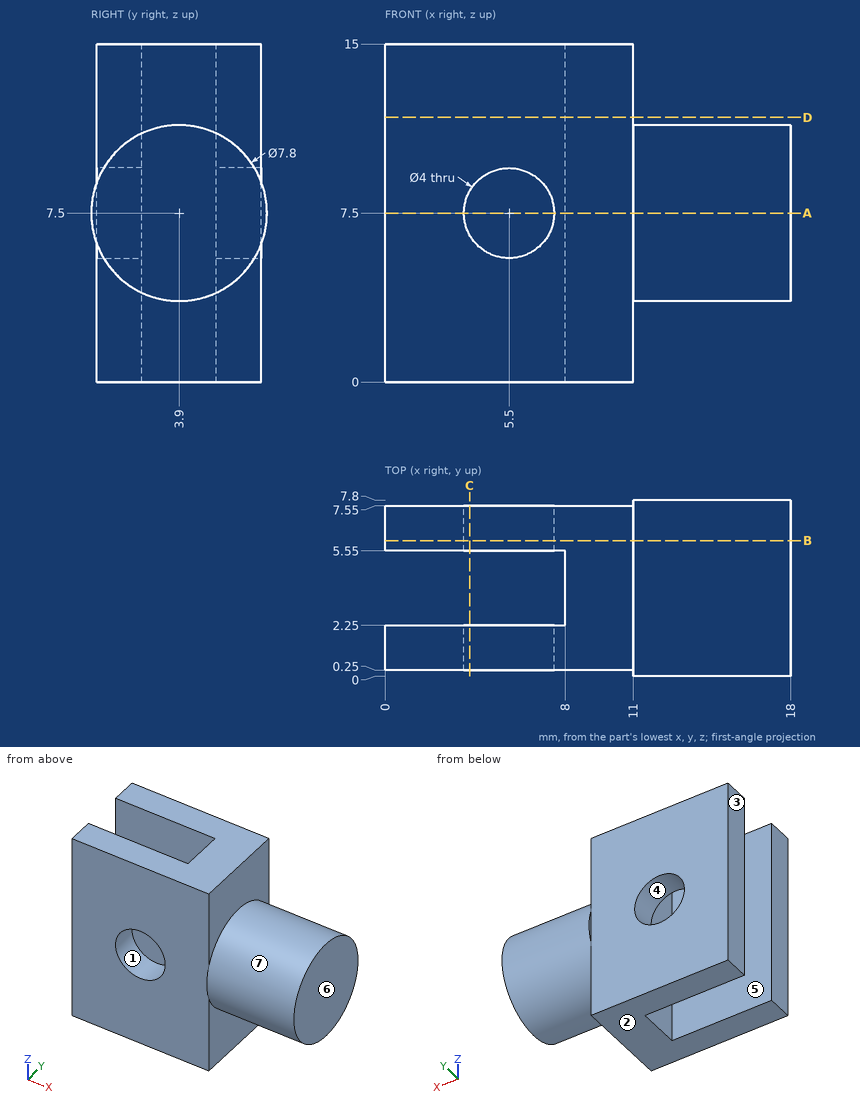
Source: three-view drawing plus pictorial views. Frame: mm from the lowest corner of the part. A direction names the side the tool comes from. Coordinates: 2 decimals unless noted, no trailing zeros. Order: outer loops, then holes, each group sorted by start corner. A loop starts at its lowest first (then second) coordinate and runs counter-clockwise, first axis right, second up. Notation, with made-up numbers: M 69.5,47 L 75.5,47 A16 cw 75.5,78 Z; hole C 3.5,85.5 d3. An arc over 180 degrees is marked long. One line per question, with ' | ' between items. Start each with the question number.
Item 1: Ray query, probe 1 along X at (y, z) = (7.05, 7.5); probe 2 along Y at (x, z) = (5.5, 4.75); probe 3 along X at (y, z) = (7, 1.25). Return the intervals inside material, ascending. Write a range as [from, to].
Item 2: Set-up query: the marked faces 5, 6 and 7. Return all of +Z, -Z, +X, -X, +Y, -Y with unobstructed straight access to the full face (end or side cutting, diameter ignored); none if empty.
Item 3: Cut plane C-C, the plane x = 3.75. Return the cut outline in (y, z), then the cut area to 3 significant figures.
Item 4: Pin query (flat end, axial travel): pin 1 Ø5.5 at (x, z) = (5.5, 11) entering from -Y; pin 2 Ø1.6 at (y, z) = (3.5, 5) entering from -X; pin 3 Ø4.5 at (x, z) = (5.5, 7.5) entering from +Y. Return the tip coordinate at first contact, or that it passes through.
Item 5: Cut plane A-A, the plane z = 7.5. Return the cut outline in (x, y), then the cut area to 3 significant figures.
Item 6: Cut plane D-D, the plane z = 11.75. Return the cut outline in (x, y), then the cut area to 3 significant figures.
Item 7: Draft query along Z for the marked faces 1, 2, 3 and 4. Return one class per face: released by +Z, released by -Z, zero draft, split by the parting line, or undercut.
Item 8: Cut plane B-B, the plane y = 6. Return the cut outline in (x, z), then the cut area to 3 significant figures.
A:
1) probe 1: x = [0, 3.5], [7.5, 18] | probe 2: y = [0.25, 2.25], [5.55, 7.55] | probe 3: x = [0, 11]
2) face 5: +Z, -Z, -X | face 6: +Z, -Z, +X, +Y, -Y | face 7: +X
3) outline: M 0.25,0 L 2.25,0 L 2.25,6.53 L 0.25,6.53 Z; M 0.25,8.47 L 2.25,8.47 L 2.25,15 L 0.25,15 Z; M 5.55,0 L 7.55,0 L 7.55,6.53 L 5.55,6.53 Z; M 5.55,8.47 L 7.55,8.47 L 7.55,15 L 5.55,15 Z | area: 52.3 mm2
4) pin 1: stops at y = 0.25 | pin 2: stops at x = 8 | pin 3: stops at y = 7.55
5) outline: M 0,0.25 L 3.5,0.25 L 3.5,2.25 L 0,2.25 Z; M 0,5.55 L 3.5,5.55 L 3.5,7.55 L 0,7.55 Z; M 7.5,0.25 L 11,0.25 L 11,0 L 18,0 L 18,7.8 L 11,7.8 L 11,7.55 L 7.5,7.55 L 7.5,5.55 L 8,5.55 L 8,2.25 L 7.5,2.25 Z | area: 92.5 mm2
6) outline: M 0,0.25 L 11,0.25 L 11,7.55 L 0,7.55 L 0,5.55 L 8,5.55 L 8,2.25 L 0,2.25 Z | area: 53.9 mm2
7) face 1: undercut | face 2: released by -Z | face 3: zero draft | face 4: undercut
8) outline: M 0,0 L 11,0 L 11,4.21 L 18,4.21 L 18,10.79 L 11,10.79 L 11,15 L 0,15 Z; hole C 5.5,7.5 d4 | area: 198 mm2
